Check sheet for the modelled part. Datum: model origin and axes. Units: mm. Face numbers are marked on the shaded views. Give positions to 0.01 mm unless a question says otherwise; leave off trailing zeros. Order: outer loops, then holes, each group sorted by start corner. A loop starts at its lowest first (then second) coordinate and runs counter-clockwise, first axis right, second up.
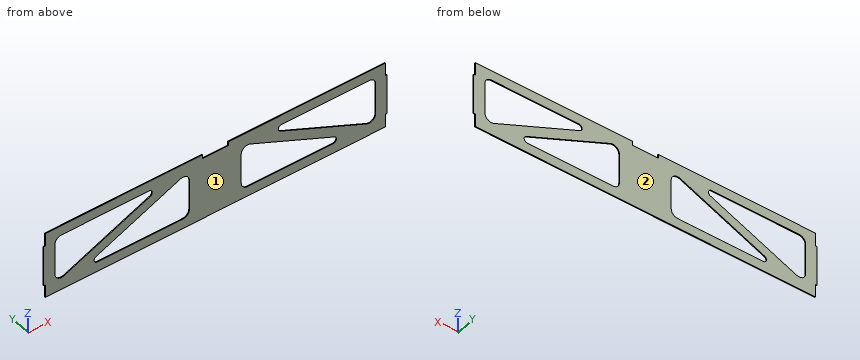
```python
from build123d import *

# Parameters (mm, degrees)
BOSS_EXTRUDE1_DEPTH = 1.5875
CUT_EXTRUDE2_DEPTH  = 343.657797193
WING_SPAR_CUT_W     = 50.8
WING_SPAR_CUT_H     = 7.62
CUT_EXTRUDE3_DEPTH  = 343.657797193


with BuildPart() as part:
    # Sketch1 → Boss-Extrude1 (new body)
    with BuildSketch(Plane(origin=(0, 0, 0), x_dir=(1, 0, 0), z_dir=(0, 1, 0))):
        Polygon((-333.375, 38.989), (-333.375, 64.389), (333.375, 64.389), (333.375, 38.989), (336.55, 38.989), (336.55, -38.989), (333.375, -38.989), (333.375, -64.389), (-333.375, -64.389), (-333.375, -38.989), (-336.55, -38.989), (-336.55, 38.989), align=None)
    extrude(amount=BOSS_EXTRUDE1_DEPTH)

    # Sketch3 → Cut-Extrude2 (cut, through all)
    with BuildSketch(Plane(origin=(0, 1.5875, 0), x_dir=(1, 0, 0), z_dir=(0, 1, 0))):
        with BuildLine():
            Line((-314.325, 27.760799149), (-314.325, -32.639))
            ThreePointArc((-314.325, -32.639), (-310.605256121, -41.619256121), (-301.625, -45.339))
            Line((-301.625, -45.339), (-129.997745545, -45.339))
            ThreePointArc((-129.997745545, -45.339), (-123.777758329, -40.267381409), (-127.49333105, -33.153727253))
            Line((-127.49333105, -33.153727253), (-296.616171009, 39.431344643))
            ThreePointArc((-296.616171009, 39.431344643), (-308.613485953, 38.365093755), (-314.325, 27.760799149))
        make_face()
        with BuildLine():
            Line((-231.183231716, 45.339), (-63.5, 45.339))
            ThreePointArc((-63.5, 45.339), (-54.519743879, 41.619256121), (-50.8, 32.639))
            Line((-50.8, 32.639), (-50.8, -26.068081748))
            ThreePointArc((-50.8, -26.068081748), (-56.511514047, -36.672376354), (-68.508828991, -37.738627243))
            Line((-68.508828991, -37.738627243), (-233.687646211, 33.153727253))
            ThreePointArc((-233.687646211, 33.153727253), (-237.403218932, 40.267381409), (-231.183231716, 45.339))
        make_face()
        with BuildLine():
            Line((68.508828991, -37.738627243), (233.687646211, 33.153727253))
            ThreePointArc((233.687646211, 33.153727253), (237.403218932, 40.267381409), (231.183231716, 45.339))
            Line((231.183231716, 45.339), (63.5, 45.339))
            ThreePointArc((63.5, 45.339), (54.519743879, 41.619256121), (50.8, 32.639))
            Line((50.8, 32.639), (50.8, -26.068081748))
            ThreePointArc((50.8, -26.068081748), (56.511514047, -36.672376354), (68.508828991, -37.738627243))
        make_face()
        with BuildLine():
            Line((314.325, 27.760799149), (314.325, -32.639))
            ThreePointArc((314.325, -32.639), (310.605256121, -41.619256121), (301.625, -45.339))
            Line((301.625, -45.339), (129.997745545, -45.339))
            ThreePointArc((129.997745545, -45.339), (123.777758329, -40.267381409), (127.49333105, -33.153727253))
            Line((127.49333105, -33.153727253), (296.616171009, 39.431344643))
            ThreePointArc((296.616171009, 39.431344643), (308.613485953, 38.365093755), (314.325, 27.760799149))
        make_face()
    extrude(amount=-CUT_EXTRUDE2_DEPTH, mode=Mode.SUBTRACT)

    # Wing Spar Cut → Cut-Extrude3 (cut, through all)
    with BuildSketch(Plane(origin=(0, 1.5875, 0), x_dir=(1, 0, 0), z_dir=(0, 1, 0))):
        with Locations((0, -60.579)):
            Rectangle(WING_SPAR_CUT_W, WING_SPAR_CUT_H)
    extrude(amount=-CUT_EXTRUDE3_DEPTH, mode=Mode.SUBTRACT)


solid = part.part
```
(1) Sectioned sample at B-B (z = 11). Count the separate pieces of the cut face and the enclosed holes in it, plus the area to 3 significant figures.
(2) Sectioned sample at C-C (x = 152.5). Enter the section's corners in (y, z), plus the area to 3 significant figures.
(3) Go/stop test with flat-tipped pins: P1, Ø0.5, axis at y = 1, z = 61.5, coming from the -X side (3 decimals); P2, Ø0.5, axis at x = 334.5, y = 0.5, coming from the -Z side; P3, Ø0.5, axis at x = -335, y = 1, coming from the +Z side. Record where each tip stops, or that it passes through.
(4) Sectioned sample at A-A (x = 272). Enter the section's corners in (y, z).
(5) Release check for a two-part mould opening along Y. For the marked faces 1 and 2 record: released by +Y, released by -Y, zero draft, split by the parting line, or undercut.
(6) Thickness scan on L1, parallel to Z at x = -129, y = 0.55; L2, parallel to X at y = 1.1, z = 6 (3 decimals); L3, parallel to X at y = 1.45, z = 37. Record the ranges inside material, lowest first.
Values follow:
1. separate pieces: 5
1. enclosed holes: 0
1. area: 385 mm2
2. outline: (0, -64.39) - (1.59, -64.39) - (1.59, -45.34) - (0, -45.34) - close; (0, 1.69) - (1.59, 1.69) - (1.59, 22.42) - (0, 22.42) - close; (0, 45.34) - (1.59, 45.34) - (1.59, 64.39) - (0, 64.39) - close
2. area: 93.4 mm2
3. P1: stops at x = -333.375
3. P2: stops at z = -38.99
3. P3: stops at z = 38.99
4. outline: (0, -64.39) - (1.59, -64.39) - (1.59, -28.87) - (0, -28.87) - close; (0, 45.34) - (1.59, 45.34) - (1.59, 64.39) - (0, 64.39) - close
5. face 1: released by -Y
5. face 2: released by +Y
6. L1: z = -64.39 to -45.34, 11.78 to 32.51, 45.26 to 64.39
6. L2: x = -336.55 to -314.325, -190.761 to -142.46, -50.8 to 50.8, 142.46 to 190.761, 314.325 to 336.55
6. L3: x = -336.55 to -313.55, -123.97 to -70.23, -57.04 to 57.04, 70.23 to 123.97, 313.55 to 336.55
